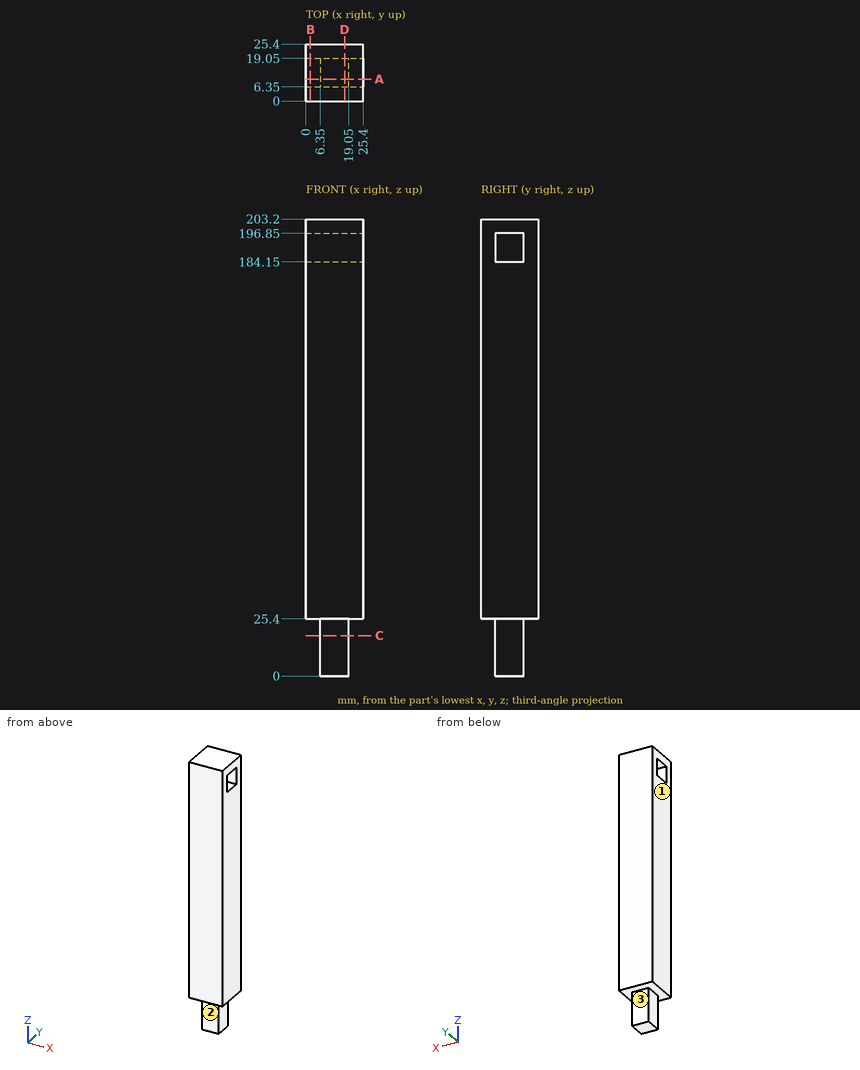
Source: three-view drawing plus pictorial views. Frame: mm from the lowest corner of the part. A direction names the side the tool comes from. Round coordinates to 2 decimals unless told otherwise and drop trailing zeros. Write each loop counter-clockwise with the first axis right and the second up, starting at its lowest first coordinate (ties: lowest second). Pieces come first, ordered by that corner, then holes. Notation, with made-up numbers: M 43.5,-32.75 L 78.5,-32.75 A6 cw 78.5,-27.75 Z; hole C -4.5,45.25 d8. An arc over 180 degrees is marked long. One line per item, written item: value. Start each with the question number.
Item 1: Pin query (flat end, axial travel): pin 1 (6.5 mm diameter, centred on x = 10, z = 15.5, fed in from +Y); pin 2 (14 mm diameter, centred on y = 11.5, z = 9, fed in from +X); pin 3 (14 mm diameter, centred on y = 10, z = 9.5, fed in from -X). Return the tip coordinate at first contact, or that it passes through.
Item 2: Ray query, L1, parallel to Z at x = 3.25, y = 13.5; L2, parallel to Y at x = 2.25, z = 189; L3, parallel to Z at x = 7.5, y = 9. Return the intervals inside material, ascending. Write a range as from..to.
Item 3: Section query A-A (y = 9.75). Return the cut outline in (x, z), plus the area to 3 significant figures.
Item 4: Set-up query: the marked faces 1, 2 and 3. Return all of +Z, -Z, +X, -X, +Y, -Y with unobstructed straight access to the full face (end or side cutting, diameter ignored); none if empty.
Item 5: Section query B-B (x = 2). Return the cut outline in (y, z), plus the area to 3 significant figures.
Item 6: Section query C-C (z = 18). Return the cut outline in (x, y).
Item 7: Section query D-D (x = 17.25). Return the cut outline in (y, z), plus the area to 3 significant figures.
Result set:
1. pin 1: stops at y = 19.05
1. pin 2: stops at x = 19.05
1. pin 3: stops at x = 6.35
2. L1: z = 25.4..184.15, 196.85..203.2
2. L2: y = 0..6.35, 19.05..25.4
2. L3: z = 0..184.15, 196.85..203.2
3. outline: M 0,25.4 L 6.35,25.4 L 6.35,0 L 19.05,0 L 19.05,25.4 L 25.4,25.4 L 25.4,184.15 L 0,184.15 Z; M 0,196.85 L 25.4,196.85 L 25.4,203.2 L 0,203.2 Z
3. area: 4,520 mm²
4. face 1: +Z, -Z, -X, +Y, -Y
4. face 2: -Z, +X, -X, -Y
4. face 3: -Z, +X, -X, +Y
5. outline: M 0,25.4 L 25.4,25.4 L 25.4,203.2 L 0,203.2 Z; hole M 6.35,184.15 L 19.05,184.15 L 19.05,196.85 L 6.35,196.85 Z
5. area: 4,350 mm²
6. outline: M 6.35,6.35 L 19.05,6.35 L 19.05,19.05 L 6.35,19.05 Z
7. outline: M 0,25.4 L 6.35,25.4 L 6.35,0 L 19.05,0 L 19.05,25.4 L 25.4,25.4 L 25.4,203.2 L 0,203.2 Z; hole M 6.35,184.15 L 19.05,184.15 L 19.05,196.85 L 6.35,196.85 Z
7. area: 4,680 mm²
